```python
from build123d import *

# Parameters (mm, degrees)
F1_DEPTH  = 22.352
F2_DEPTH  = 3.175
F4_R      = 22.35199
F5_R      = 3.175
F6_DEPTH  = 25.4
F7_R      = 6.35
F7_R_2    = 3.175
F8_DEPTH  = 3.175
F9_R      = 10.922
F10_DEPTH = 25.4


# Not quite as in the source:
# - a fillet or chamfer is up to 0.001 mm smaller than in the source, because OpenCascade refuses the exact size


with BuildPart() as f1:
    # F0 (on Front) → F1 (new body, symmetric)
    with BuildSketch(Plane.XZ):
        Polygon((-3.9430456236, 0), (-29.3430456236, 0), (-48.3930456236, 32.9955678842), (-56.7519228209, 28.1695678842), (-34.9156304218, -9.652), (56.8391502193, -9.652), (56.5089543764, 0), align=None)
    extrude(amount=F1_DEPTH, both=True)

    # F0 (on Front) → F2 (join, symmetric)
    with BuildSketch(Plane.XZ):
        Polygon((-48.3930456236, 32.9955678842), (-29.3430456236, 0), (-3.9430456236, 0), align=None)
    extrude(amount=F2_DEPTH, both=True)

    # F4 (radius 22.352 in the source; OpenCascade refuses exactly that, so slightly less here)
    f4_edges = [f1.edges().sort_by_distance(p)[0] for p in [
        (56.674052, -22.352, -4.826),
        (56.674052, 22.352, -4.826),
    ]]
    fillet(f4_edges, radius=F4_R)

    # F5 (on face) → F6 (cut)
    with BuildSketch(Plane(origin=(-30.366161415, 0, -17.5319114672), x_dir=(0, -1, 0), z_dir=(-0.8660254038, 0, -0.5))):
        with Locations((-11.43, 41.8495228118)):
            Circle(F5_R)
        with Locations((12.2398376594, 41.8495228118)):
            Circle(F5_R)
    extrude(amount=-F6_DEPTH, mode=Mode.SUBTRACT)

    # F7 (on face) → F8 (cut)
    with BuildSketch(Plane(origin=(-22.0072842177, 0, -12.7059114672), x_dir=(0, 1, 0), z_dir=(0.8660254038, 0, 0.5))):
        with Locations((-12.2398376594, 41.8495228118)):
            Circle(F7_R)
        with Locations((-12.2398376594, 41.8495228118)):
            Circle(F7_R_2, mode=Mode.SUBTRACT)
        with Locations((11.43, 41.8495228118)):
            Circle(F7_R)
    extrude(amount=-F8_DEPTH, mode=Mode.SUBTRACT)

    # F9
    f9_edges = [f1.edges().sort_by_distance(p)[0] for p in [
        (-52.572484, 22.352, 30.582568),
        (-52.572484, -22.352, 30.582568),
    ]]
    fillet(f9_edges, radius=F9_R)

    # F3 (on face) → F10 (cut)
    with BuildSketch(Plane.XY):
        with BuildLine():
            Line((37.2716346684, 9.027880175), (11.8716346684, 9.027880175))
            ThreePointArc((11.8716346684, 9.027880175), (2.8515551479, -0.6319204795), (12.5113558024, -9.652))
            Line((12.5113558024, -9.652), (37.9113558024, -9.652))
            ThreePointArc((37.9113558024, -9.652), (44.825892917, -0.0643068731), (37.2716346684, 9.027880175))
        make_face()
    extrude(amount=-F10_DEPTH, mode=Mode.SUBTRACT)


solid = f1.part
```
Could you check a few things on this model? Use its own coordinates, in mm. A direction names the side the tool comes from. Give positions to 0.01 mm unless a question says otherwise; leave off trailing zeros. Order: outer loops, then holes, each group sorted by start corner. A loop starts at its lowest first (then second) coordinate and runs counter-clockwise, first axis right, second up.
Q1. I'm going to push flat-ended pins straight in: P1, Ø8, axis at y = -4, z = -1.5, coming from the +X side; P2, Ø3, axis at y = 9, z = 25.5, coming from the -X side; P3, Ø22.5, axis at x = -4, y = -9, coming from the +Z side. Where does each tip first touch, or does it pass through?
Q2. Suppose I cut it at B-B, the plane y = 7. Write out the boundary of the cut face in (x, z).
Q3. We'd pull the mould along Y, two halves only. Please class faces 1 (the flat face through (0, 0, -9.652)), 2 (the cylindrical face through (50.29, -15.63, -4.59)), 3 (the cylindrical face through (44.83, -0.24, -4.76)), 4 (the flat face through (-44.315, -9.507, 19.582)): +Y half, -Y half, draft (parallel to the pull), parting line (faces both ways), or undercut.
Q4. Suppose I cut it at C-C, the plane z = 11.5. Write out the boundary of the cut face in (x, y) (3 decimals).
Q5. Suppose I cut it at A-A, the plane x = 6.5. Write out the boundary of the cut face in (y, z), and give its area (3 significant figures).
Q6. For faces 5 (the flat face through (14, 10, 0)), 6 (the flat face through (-36.618, 12.629, 12.601)), 7 (the cylindrical face through (2.847, -0.426, -4.758)), 8 (the flat face through (-36.618, -12.898, 12.601)), which set-ups out of +Z, -Z, +X, -X, +Y, -Y let a thin tool reach every point of the face, with its end or its side?
Q7. If I drill on line 1 along Y through (x, z) = (-25.5, 6) (3 decimals); line 2 along Z through (x, y) = (3, -5); line 3 along Z through (x, y) = (-31, -13), over which ranges is the centre line in solid material (lowest first)?
Q8. Suppose I cut it at D-D, the plane x = -5. Write out the boundary of the cut face in (y, z) (3 decimals).
Solution:
1. P1: stops at x = 56.63
1. P2: stops at x = -56.08
1. P3: stops at z = 7.19
2. outline: (-56.75, 28.17) - (-34.92, -9.65) - (6.37, -9.65) - (6.37, 0) - (-29.34, 0) - (-40.66, 19.6) - (-43.41, 18.01) - (-47.96, 25.89) - (-45.21, 27.48) - (-48.39, 33) - close; (41.38, -9.65) - (55.71, -9.65) - (55.38, 0) - (41.38, 0) - close
3. face 1: draft
3. face 2: -Y half
3. face 3: undercut
3. face 4: undercut
4. outline: (-47.128, -22.352) - (-35.983, -22.352) - (-35.983, -3.175) - (-19.435, -3.175) - (-19.435, 3.175) - (-35.983, 3.175) - (-35.983, 22.352) - (-47.128, 22.352) - close
5. outline: (-22.35, -9.65) - (-7.72, -9.65) - (-7.72, 0) - (-22.35, 0) - close; (7.1, -9.65) - (22.35, -9.65) - (22.35, 0) - (7.1, 0) - close
5. area: 288 mm2
6. face 5: +Z, +X
6. face 6: +Z, +X, +Y
6. face 7: +Z, -Z
6. face 8: +Z, +X, -Y
7. line 1: y = -3.175 to 3.175
7. line 2: z = -9.65 to 0
7. line 3: z = -9.65 to 2.87
8. outline: (-22.352, -9.652) - (22.352, -9.652) - (22.352, 0) - (3.175, 0) - (3.175, 0.785) - (-3.175, 0.785) - (-3.175, 0) - (-22.352, 0) - close
